Can you work these out from the model? Positions are in its coordinate system, mm. A direction names the side the tool comes from. Give positions to 0.01 mm unless a question says otherwise; leave off trailing zeros. Write each loop counter-clockwise with the first axis right and the second up, starting at its lowest first coordinate (ties: lowest second). Pieces come first, ordered by that corner, then holes.
from build123d import *

# Parameters (mm, degrees)
SKETCH_1_R      = 5
SKETCH_1_R_2    = 2.75
EXTRUDE_1_DEPTH = 10


with BuildPart() as part:
    # 草图1 → 凸台-拉伸1 (new body)
    # profile 1 of 5: a face of its own
    with BuildSketch(Plane.XY):
        with BuildLine():
            ThreePointArc((3.125, 9.499177596), (0, 10), (-3.125, 9.499177596))
            ThreePointArc((-3.125, 9.499177596), (-9.91048591, -1.335016492), (-0.5, -9.987492178))
            Line((-0.5, -9.987492178), (-0.5, -7.481214682))
            Line((-0.5, -7.481214682), (-0.5, -4.974937186))
            ThreePointArc((-0.5, -4.974937186), (-3.354101966, 3.708099244), (5, 0))
            ThreePointArc((5, 0), (3.708099244, -3.354101966), (0.5, -4.974937186))
            Line((0.5, -4.974937186), (0.5, -7.481214682))
            Line((0.5, -7.481214682), (0.5, -9.987492178))
            ThreePointArc((0.5, -9.987492178), (7.245688373, -6.892024376), (10, 0))
            ThreePointArc((10, 0), (8.100925873, 5.8630197), (3.125, 9.499177596))
        make_face()
    # profile 2 of 5: a face of its own
    with BuildSketch(Plane.XY):
        with BuildLine():
            Line((-3.125, 9.499177596), (-17.5625, 4.749588798))
            ThreePointArc((-17.5625, 4.749588798), (-13.06849015, 4.050462937), (-11, 0))
            ThreePointArc((-11, 0), (-13.010355295, -4.007745568), (-17.424809815, -4.792694127))
            Line((-17.424809815, -4.792694127), (-10, -7))
            Line((-10, -7), (-10, -14))
            Line((-10, -14), (-0.5, -14))
            Line((-0.5, -14), (-0.5, -9.987492178))
            ThreePointArc((-0.5, -9.987492178), (-9.91048591, -1.335016492), (-3.125, 9.499177596))
        make_face()
    # profile 3 of 5: a face of its own
    with BuildSketch(Plane.XY):
        with Locations((-16, 0)):
            Circle(SKETCH_1_R)
        with Locations((-16, 0)):
            Circle(SKETCH_1_R_2, mode=Mode.SUBTRACT)
    # profile 4 of 5: a face of its own
    with BuildSketch(Plane.XY):
        with BuildLine():
            Line((17.5625, 4.749588798), (3.125, 9.499177596))
            ThreePointArc((3.125, 9.499177596), (8.100925873, 5.8630197), (10, 0))
            ThreePointArc((10, 0), (7.245688373, -6.892024376), (0.5, -9.987492178))
            Line((0.5, -9.987492178), (0.5, -14))
            Line((0.5, -14), (10, -14))
            Line((10, -14), (10, -7))
            Line((10, -7), (17.424809815, -4.792694127))
            ThreePointArc((17.424809815, -4.792694127), (11.000520443, 0.072139893), (17.5625, 4.749588798))
        make_face()
    # profile 5 of 5: a face of its own
    with BuildSketch(Plane.XY):
        with Locations((16, 0)):
            Circle(SKETCH_1_R)
        with Locations((16, 0)):
            Circle(SKETCH_1_R_2, mode=Mode.SUBTRACT)
    extrude(amount=EXTRUDE_1_DEPTH)


solid = part.part
(1) Imagine slicing it at A-A, the plane z = 2. Give the number of separate pieces and of enclosed holes in the cut face, plus the area to 3 significant figures.
Returned:
separate pieces: 1
enclosed holes: 2
area: 549 mm2
(2) If I drill on L1, parallel to X at y = -2.25, z = 1.75; L2, parallel to X at y = -2, z = 4.25; L3, parallel to Y at x = -16, z = 2.25, over which ranges is the centre line in solid material (lowest first)?
Returned:
L1: x = -20.47 to -17.58, -14.42 to -4.47, 4.47 to 14.42, 17.58 to 20.47
L2: x = -20.58 to -17.89, -14.11 to -4.58, 4.58 to 14.11, 17.89 to 20.58
L3: y = -5.22 to -2.75, 2.75 to 5.26
(3) Imagine slicing it at D-D, the plane y = -3.75. Write out the boundary of the cut face in (x, z), plus the area to 3 significant figures.
Returned:
outline: (-19.31, 0) - (-3.31, 0) - (-3.31, 10) - (-19.31, 10) - close; (3.31, 0) - (19.31, 0) - (19.31, 10) - (3.31, 10) - close
area: 320 mm2
(4) Will these pins go through, and if not, where does the flat tip stop? P1, Ø5.5, axis at y = -11.5, z = 3.5, coming from the -X side; P2, Ø2.5, axis at y = -11, z = 4, coming from the +X side.
Returned:
P1: stops at x = -10
P2: stops at x = 10
(5) For faces 1 (the face through (-10, -10, 5)), 2 (the face through (13.253, 0.121, 4.93)), 3 (the face through (-0.5, -10, 5)), 4 (the face through (10, -11, 5)), which set-ups out of +Z, -Z, +X, -X, +Y, -Y let a thin tool reach every point of the face, with its end or its side?
Returned:
face 1: +Z, -Z, -X, -Y
face 2: +Z, -Z
face 3: +Z, -Z, -Y
face 4: +Z, -Z, +X, -Y
(6) Imagine slicing it at C-C, the plane y = -0.75. Write out the boundary of the cut face in (x, z), plus the area to 3 significant figures.
Returned:
outline: (-20.94, 0) - (-18.65, 0) - (-18.65, 10) - (-20.94, 10) - close; (-13.35, 0) - (-4.94, 0) - (-4.94, 10) - (-13.35, 10) - close; (4.94, 0) - (13.35, 0) - (13.35, 10) - (4.94, 10) - close; (18.65, 0) - (20.94, 0) - (20.94, 10) - (18.65, 10) - close
area: 214 mm2
(7) Imagine slicing it at B-B, the plane x = 16. Write out the boundary of the cut face in (y, z), plus the area to 3 significant figures.
Returned:
outline: (-5.22, 0) - (-2.75, 0) - (-2.75, 10) - (-5.22, 10) - close; (2.75, 0) - (5.26, 0) - (5.26, 10) - (2.75, 10) - close
area: 49.8 mm2
(8) If we mould it in two halves opening along X, with no side actions, what happens to faces 5 (the face through (-5, -2, 10)), 6 (the face through (0.5, -9, 5)), 7 (the face through (21, 0, 5)), 8 (the face through (-18.747, 0.121, 4.93))? For each: +X half, -X half, draft (parallel to the pull), parting line (faces both ways), or undercut.
Returned:
face 5: draft
face 6: undercut
face 7: +X half
face 8: undercut
